from build123d import *

# Parameters (mm, degrees)
ESBO_O1_R                = 3
RESSALTO_EXTRUS_O1_DEPTH = 4


with BuildPart() as part:
    # Esboço1 → Ressalto-extrusão1 (new body)
    with BuildSketch(Plane.XY):
        with BuildLine():
            Line((-8.209602621, 0), (8.209602621, 0))
            Line((8.209602621, 0), (13, 0))
            Line((13, 0), (13, 2.609213558))
            Line((13, 2.609213558), (7.613786386, 2.609213558))
            Line((7.613786386, 2.609213558), (5.849431135, 10.335722798))
            ThreePointArc((5.849431135, 10.335722798), (0, 15), (-5.849431135, 10.335722798))
            Line((-5.849431135, 10.335722798), (-7.613786386, 2.609213558))
            Line((-7.613786386, 2.609213558), (-13, 2.609213558))
            Line((-13, 2.609213558), (-13, 0))
            Line((-13, 0), (-8.209602621, 0))
        make_face()
        with Locations((0, 9)):
            Circle(ESBO_O1_R, mode=Mode.SUBTRACT)
    extrude(amount=RESSALTO_EXTRUS_O1_DEPTH)


solid = part.part
Build history of the part. All positions in model axes, mm. A direction names the side the tool comes from. Round coordinates to 2 decimals unless told otherwise and drop trailing zeros. Write each loop counter-clockwise with the first axis right and the second up, starting at its lowest first coordinate (ties: lowest second). Pieces come first, ordered by that corner, then holes. Notation, with made-up numbers: (16, 34) -> (75, 34) arc R18 ccw to (75, 38) -> close; hole circle Ø2 at (0, -40). An arc over 180 degrees is marked (long way). Use one line per item in the form item = value.
Q1. Drop flat-ended pins along their axis: P1, Ø1.5, axis at y = 12, z = 2, coming from the -X side; P2, Ø1, axis at x = 8.5, z = 3, coming from the +Y side; P3, Ø1.5, axis at y = 10.5, z = 2, coming from the +X side. Give the stop position or say it passes through.
Conclusion:
P1 = -5.56
P2 = 2.61
P3 = 5.98
Q2. Band-saw the part on D-D, the plane x = -9.25. Write the cut outline in (y, z).
Conclusion:
outline = (0, 0) -> (2.61, 0) -> (2.61, 4) -> (0, 4) -> close
Q3. Band-saw the part on A-A, the plane z = 3.55. Write the cut outline in (x, y), then the cut area to 3 significant figures.
Conclusion:
outline = (-13, 0) -> (13, 0) -> (13, 2.61) -> (7.61, 2.61) -> (5.85, 10.34) arc R6 ccw to (-5.85, 10.34) -> (-7.61, 2.61) -> (-13, 2.61) -> close; hole circle Ø6 at (0, 9)
area = 184 mm²
Q4. Tool access for faces 1 (the flat face through (-10, 2.609, 2)), 2 (the flat face through (0, 0, 2)), 3 (the flat face through (10, 2.609, 2)): list every direction of +Z, -Z, +X, -X, +Y, -Y with a clear straight run to the whole face (end or side of a thin tool).
Conclusion:
face_1 = +Z, -Z, -X, +Y
face_2 = +Z, -Z, +X, -X, -Y
face_3 = +Z, -Z, +X, +Y
Q5. Band-saw the part on C-C, the plane y = 7.25. Write the cut outline in (x, z), then the cut area to 3 significant figures.
Conclusion:
outline = (-6.55, 0) -> (-2.44, 0) -> (-2.44, 4) -> (-6.55, 4) -> close; (2.44, 0) -> (6.55, 0) -> (6.55, 4) -> (2.44, 4) -> close
area = 32.9 mm²
Q6. Band-saw the part on B-B, the plane x = 0. Write the cut outline in (y, z).
Conclusion:
outline = (0, 0) -> (6, 0) -> (6, 4) -> (0, 4) -> close; (12, 0) -> (15, 0) -> (15, 4) -> (12, 4) -> close
Q7. Drill centre lines: L1, parallel to Y at x = 0, z = 1.25; L2, parallel to Y at x = 11.5, z = 0.35; L3, parallel to Y at x = 2, z = 0.35. Where is each one in solid material? Low to high.
Conclusion:
L1 = 0 to 6, 12 to 15
L2 = 0 to 2.61
L3 = 0 to 6.76, 11.24 to 14.66
Q8. Two-plate mould, pull along Y, no slides. Class faces 4 (the cylindrical face through (-3, 9, 2)), 5 (the cylindrical face through (0, 15, 2)), 6 (the flat face through (13, 1, 2)): released by +Y, released by -Y, zero draft, split by the parting line, or undercut.
Conclusion:
face_4 = undercut
face_5 = released by +Y
face_6 = zero draft
